For this review, take the finished solid that the model builds, in its own axes (mm). Round coordinates to 2 decimals unless told otherwise and drop trailing zeros. Loops run counter-clockwise (first coordinate to the right, second up) from the corner with the lowest first, then second, coordinate; pieces in that order, holes last.
1. Consider section A-A on x = 0. State the section outline as (y, z) points (3 decimals).
2. Clearance check with flat-ended pins moving along their axes: pin 1 Ø2 at (x, z) = (1.5, 1) entering from +Y; pin 2 Ø2 at (y, z) = (-9.5, 1.5) entering from +X; pin 3 Ø1 at (y, z) = (-12.5, 2) entering from -X. State where each tip first meets the part, or that it passes through.
3. Draft analysis for pull direction X (two halves, no side actions). For faces 1 (the cylindrical face through (-8.43, -6.47, 2.97)), 2 (the cylindrical face through (-5.961, -26.846, 2.718)), 3 (the cylindrical face through (-16, 0, 3)), 4 (the flat face through (12, 0, 0)), state which applies: released by +X, released by -X, zero draft, split by the parting line, or undercut.
4. Consider section B-B on z = 4.15. State the section outline as (x, y) points (3 decimals), then the cut area to 3 significant figures.
5. To check wall thickness, follow line 1 along Y through (x, z) = (0, 2.3) (3 decimals); line 2 along Y through (x, z) = (19, 2.8); line 3 along X through (y, z) = (-0.5, 4.55). State the ranges of each line that lie inside material, in increasing order.
from build123d import *

# Parameters (mm, degrees)
SKETCH_R         = 27.5
SKETCH_R_2       = 10.625
PAD_DEPTH        = 5
CHAMFER_SIZE     = 0.5
CHAMFER001_SIZE  = 1
HOLE_D           = 6
HOLE_CSINK_D     = 8
HOLE_CSINK_ANGLE = 90


with BuildPart() as part:
    # Sketch → Pad (new body)
    with BuildSketch(Plane.XY):
        Circle(SKETCH_R)
        Circle(SKETCH_R_2, mode=Mode.SUBTRACT)
    extrude(amount=PAD_DEPTH)

    # Chamfer
    chamfer_edges = [part.edges().sort_by_distance(p)[0] for p in [
        (-27.5, 0, 0),
    ]]
    chamfer(chamfer_edges, length=CHAMFER_SIZE)

    # Chamfer001
    chamfer001_edges = [part.edges().sort_by_distance(p)[0] for p in [
        (-10.625, 0, 0),
    ]]
    chamfer(chamfer001_edges, length=CHAMFER001_SIZE)

    # Hole (through all)
    with Locations(Plane(origin=(0, 0, 0), x_dir=(1, 0, 0), z_dir=(0, 0, -1))):
        with Locations((-19, 0), (19, 0)):
            CounterSinkHole(HOLE_D / 2, HOLE_CSINK_D / 2, counter_sink_angle=HOLE_CSINK_ANGLE)


solid = part.part
Resolved:
1. outline: (-27.5, 0.5) - (-27, 0) - (-11.625, 0) - (-10.625, 1) - (-10.625, 5) - (-27.5, 5) - close; (10.625, 1) - (11.625, 0) - (27, 0) - (27.5, 0.5) - (27.5, 5) - (10.625, 5) - close
2. pin 1: stops at y = 27.5
2. pin 2: stops at x = 26.15
2. pin 3: stops at x = -24.74
3. face 1: undercut
3. face 2: split by the parting line
3. face 3: undercut
3. face 4: zero draft
4. outline: circle Ø55 at (0, 0); hole circle Ø6 at (-19, 0); hole circle Ø21.25 at (0, 0); hole circle Ø6 at (19, 0)
4. area: 1,960 mm2
5. line 1: y = -27.5 to -10.625, 10.625 to 27.5
5. line 2: y = -19.88 to -3, 3 to 19.88
5. line 3: x = -27.5 to -21.96, -16.04 to -10.61, 10.61 to 16.04, 21.96 to 27.5
